Here's how the part is built. I have some questions about the finished solid (model axes, mm). A direction names the side the tool comes from. Round coordinates to 2 decimals unless told otherwise and drop trailing zeros. Write each loop counter-clockwise with the first axis right and the second up, starting at its lowest first coordinate (ties: lowest second). Pieces come first, ordered by that corner, then holes. Notation, with made-up numbers: (18, -39.5) - (52, -39.5) arc R22 cw to (52, -31.5) - close; hole circle Ø1 at (72.25, 34.5). An arc over 180 degrees is marked (long way). One line per question, with ' | ' between items. Start each with the question number.
(1) If I drill on L1, parallel to X at y = 346, z = -86.5; L2, parallel to Z at x = 234, y = 199, over which ranges is the centre line in solid material (lowest first)?
(2) Imagine slicing it at A-A (x = 272). Write out the boundary of the cut face in (y, z), plus the area to 3 significant figures.
(3) For faces 5 (the flat face through (197, 0, -108)), 6 (the flat face through (196, 404, -310)), which set-ups out of +Z, -Z, +X, -X, +Y, -Y let a thin tool reach every point of the face, with its end or its side?
(4) Imagine slicing it at B-B (z = 29.5). Write out the boundary of the cut face in (x, y).
(5) Will this pin go through, and if not, where does the flat tip stop? pin 1 (8 mm diameter, centred on x = 148.5, y = 84.5, fed in from -Z).
(6) Thinking about a two-plate mould opening in X: for faces 1 (the flat face through (500, 196, -59)), 2 (the flat face through (-100, 196, -59)), 3 (the flat face through (196, 500, -59)), 4 (the flat face through (197, 203, 100)), which applies, pulls with the +X half, pulls with the -X half, needs draft (parallel to the pull), parting line crosses it, or undercut?
from build123d import *

# Parameters (mm, degrees)
BOX009_W     = 400
BOX009_H     = 400
BOX009_DEPTH = 410
BOX008_W     = 600
BOX008_H     = 600
BOX008_DEPTH = 510


with BuildPart() as cube008:
    # Box009 → Box009 (new body)
    with BuildSketch(Plane.XY.offset(-310)):
        with Locations((200, 200)):
            Rectangle(BOX009_W, BOX009_H)
    extrude(amount=BOX009_DEPTH)


with BuildPart() as cut004:
    # Box008 → Box008 (new body)
    with BuildSketch(Plane(origin=(-100, -100, -310), x_dir=(1, 0, 0), z_dir=(0, 0, 1))):
        with Locations((300, 300)):
            Rectangle(BOX008_W, BOX008_H)
    extrude(amount=BOX008_DEPTH)

    # Cut004: cut Cube008
    add(cube008.part, mode=Mode.SUBTRACT)


solid = cut004.part
Check sheet entries:
1) L1: -100 to 0, 400 to 500 | L2: 100 to 200
2) outline: (-100, -310) - (0, -310) - (0, 100) - (400, 100) - (400, -310) - (500, -310) - (500, 200) - (-100, 200) - close | area: 142,000 mm^2
3) face 5: -Z | face 6: -Z, +X, -X, +Y, -Y
4) outline: (-100, -100) - (500, -100) - (500, 500) - (-100, 500) - close; hole (0, 0) - (400, 0) - (400, 400) - (0, 400) - close
5) pin 1: z = 100
6) face 1: pulls with the +X half | face 2: pulls with the -X half | face 3: needs draft | face 4: undercut
